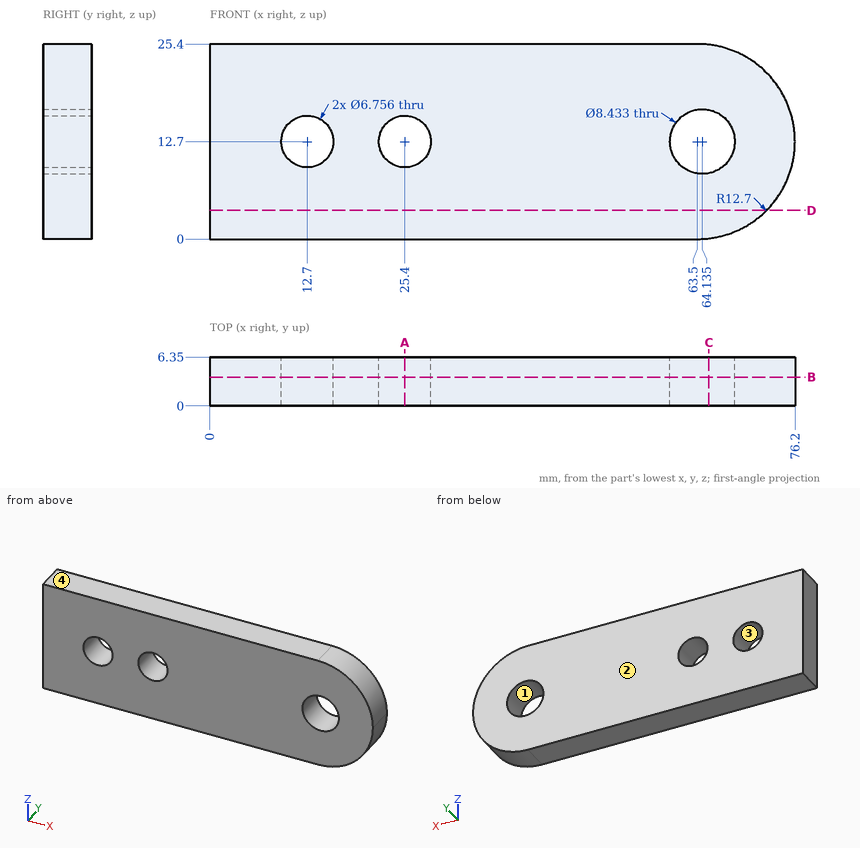
Geometry check sheet. Reference: drawing and pictorial views, mm from the part's lowest x, y, z. Round coordinates to 2 decimals unless told otherwise and drop trailing zeros. Order: outer loops, then holes, each group sorted by start corner. A loop starts at its lowest first (then second) coordinate and runs counter-clockwise, first axis right, second up. Notation, with made-up numbers: (46, 5.25) - (60, 5.25) arc R20 ccw to (60, 35.25) - close; hole circle Ø6 at (10.5, 16). An arc over 180 degrees is marked (long way). Write item = value, one per line.
Q1. Section check D-D (z = 3.75). Record the boundary of the cut face in (x, y).
Computed:
outline = (0, 0) - (72.51, 0) - (72.51, 6.35) - (0, 6.35) - close
Q2. Draft check along Z on the marked faces 1, 2, 3 and 4. Enter one of: pulls with the +Z half, pulls with the -Z half, needs draft (parallel to the pull), parting line crosses it, or undercut.
Computed:
face_1 = undercut
face_2 = needs draft
face_3 = undercut
face_4 = pulls with the +Z half
Q3. Section check A-A (x = 25.4). Record the boundary of the cut face in (y, z).
Computed:
outline = (0, 0) - (6.35, 0) - (6.35, 9.32) - (0, 9.32) - close; (0, 16.08) - (6.35, 16.08) - (6.35, 25.4) - (0, 25.4) - close
Q4. Section check B-B (y = 3.75). Record the boundary of the cut face in (x, z) (1 decimal), and give its area (3 significant figures).
Computed:
outline = (0, 0) - (63.5, 0) arc R12.7 ccw to (63.5, 25.4) - (0, 25.4) - close; hole circle Ø6.8 at (12.7, 12.7); hole circle Ø6.8 at (25.4, 12.7); hole circle Ø8.4 at (64.1, 12.7)
area = 1,740 mm^2
Q5. Go/stop test with flat-tipped pins: pin 1 (5.5 mm diameter, centred on x = 12.7, z = 12.7, fed in from +Y); pin 2 (9 mm diameter, centred on x = 25.4, z = 12.7, fed in from -Y). Record where each tip stops, or that it passes through.
Computed:
pin_1 = through
pin_2 = 0
Q6. Thickness scan on line 1 along Z through (x, y) = (25.4, 3.5); line 2 along X through (y, z) = (3.75, 10.5) (1 decimal); line 3 along Z through (x, y) = (68, 2) (1 decimal). Record the ranges inside material, lowest first.
Computed:
line_1 = 0 to 9.32, 16.08 to 25.4
line_2 = 0 to 10.1, 15.3 to 22.8, 28 to 60.5, 67.7 to 76
line_3 = 0.8 to 11, 14.4 to 24.6
Q7. Section check C-C (x = 65). Record the boundary of the cut face in (y, z), and give its area (3 significant figures).
Computed:
outline = (0, 0.09) - (6.35, 0.09) - (6.35, 8.57) - (0, 8.57) - close; (0, 16.83) - (6.35, 16.83) - (6.35, 25.31) - (0, 25.31) - close
area = 108 mm^2
